Read the model definition and answer for the solid it produces. Units are mm, in the model's axes. A direction names the side the tool comes from. Coordinates: 2 decimals unless noted, no trailing zeros. Loops run counter-clockwise (first coordinate to the right, second up) from the corner with the lowest first, then second, coordinate; pieces in that order, holes last.
from build123d import *

# Parameters (mm, degrees)
F1_DEPTH = 11.1125
F2_W     = 3.175
F2_H     = 9.525
F3_DEPTH = 9.525
F4_R     = 2.15265
F5_DEPTH = 34.925
F6_R     = 1.7272
F7_DEPTH = 4.7625


with BuildPart() as f1:
    # F0 (on Top) → F1 (new body)
    with BuildSketch(Plane.XY):
        Polygon((0, 0), (-34.925, 0), (-34.925, -30.1625), (-30.1625, -30.1625), (-30.1625, -4.7625), (-4.7625, -4.7625), (-4.7625, -30.1625), (0, -30.1625), align=None)
    extrude(amount=F1_DEPTH)

    # F2 (on face) → F3 (cut)
    with BuildSketch(Plane.XY.offset(11.1125)):
        with Locations((-31.75, -23.8125)):
            Rectangle(F2_W, F2_H)
        with Locations((-3.175, -23.8125)):
            Rectangle(F2_W, F2_H)
    extrude(amount=-F3_DEPTH, mode=Mode.SUBTRACT)

    # F4 (on face) → F5 (cut, through all)
    with BuildSketch(Plane(origin=(-34.925, 0, 0), x_dir=(0, -1, 0), z_dir=(-1, 0, 0))):
        with Locations((23.8125, 6.35)):
            Circle(F4_R)
    extrude(amount=-F5_DEPTH, mode=Mode.SUBTRACT)

    # F6 (on face) → F7 (cut, through all)
    with BuildSketch(Plane.XZ.offset(4.7625)):
        with Locations((-7.9375, 5.55625)):
            Circle(F6_R)
        with Locations((-26.9875, 5.55625)):
            Circle(F6_R)
    extrude(amount=-F7_DEPTH, mode=Mode.SUBTRACT)


solid = f1.part
Q1. Flat-ended cylindrical pins translate along their axes: pin 1 Ø5 at (x, z) = (-13.5, 2) entering from -Y; pin 2 Ø1.6 at (x, y) = (-32.5, -23) entering from +Z. Find the tip coordinate at first contact, or state that the pin passes through.
Findings below:
pin 1: stops at y = -4.76
pin 2: stops at z = 1.59
Q2. A cutting plane is placed at C-C (z = 6.35). Count the separate pieces of the cut face and the enclosed holes in it, then the cut area to 3 significant figures.
Findings below:
separate pieces: 5
enclosed holes: 0
area: 305 mm2
Q3. Straight lines are drawn through the part: probe 1 along X at (y, z) = (-11, 7.5) (1 decimal); probe 2 along X at (y, z) = (-26.5, 6.5) (1 decimal); probe 3 along Y at (x, z) = (-19, 3.25). For each, find the intervals that lie inside material, in ascending order.
Findings below:
probe 1: x = -34.9 to -30.2, -4.8 to 0
probe 2: x = -34.9 to -33.3, -1.6 to 0
probe 3: y = -4.76 to 0
Q4. Which of the six approach directions +Z, -Z, +X, -X, +Y, -Y give full straight-line access (tool end or side, diameter ignored) to faces 1 (the face through (-4.762, -12, 5)), 2 (the face through (-3, -19.05, 6)), 3 (the face through (-34.142, -22.104, 5.04))?
Findings below:
face 1: +Z, -Z, -Y
face 2: +Z
face 3: +X, -X
Q5. A cutting plane is placed at B-B (x = -26.5). Give the vertices of the cut face in (y, z).
Findings below:
outline: (-4.76, 0) - (0, 0) - (0, 3.9) - (-4.76, 3.9) - close; (-4.76, 7.21) - (0, 7.21) - (0, 11.11) - (-4.76, 11.11) - close
Q6. Determine the mould class of faces 4 (the face through (-3, -24, 1.588)), 5 (the face through (-34.925, -15, 5)), 6 (the face through (-18, -4.762, 5)), 7 (the face through (-17, 0, 5)) for opening direction Y: +Y half, -Y half, draft (parallel to the pull), parting line (faces both ways), or undercut.
Findings below:
face 4: undercut
face 5: draft
face 6: -Y half
face 7: +Y half
Q7. A cutting plane is placed at A-A (y = -17.5). Give the vertices of the cut face in (x, z) (1 decimal), then the cut area to 3 significant figures.
Findings below:
outline: (-34.9, 0) - (-30.2, 0) - (-30.2, 11.1) - (-34.9, 11.1) - close; (-4.8, 0) - (0, 0) - (0, 11.1) - (-4.8, 11.1) - close
area: 106 mm2
